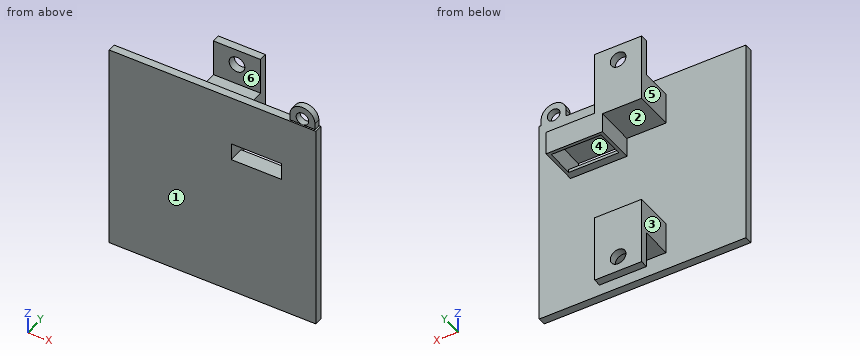
Autodesk Inventor part; units mm, degrees
ref_plane "YZ Plane" through (0, 0, 0) normal (1, 0, 0) x (0, 1, 0)
ref_plane "XZ Plane" through (0, 0, 0) normal (0, 1, 0) x (-1, 0, 0)
ref_plane "XY Plane" through (0, 0, 0) normal (0, 0, 1) x (1, 0, 0)
sketch "Szkic1" plane through (0, 0, 0) normal (0, 1, 0) x (-1, 0, 0)
  line L0 (26.7, -27.1) -> (-26.7, -27.1)
  line L1 (-26.7, -27.1) -> (-26.7, 27.1)
  line L2 (-26.7, 27.1) -> (26.7, 27.1)
  line L3 (26.7, 27.1) -> (26.7, -27.1)
  line L4 (26.7, -27.1) -> (-26.7, 27.1) construction
  line L5 (-26.7, -27.1) -> (26.7, 27.1) construction
  point P0 (0, 0)
  dimension "d0" = 53.4
  dimension "d1" = 54.2
extrude "Wyciągnięcie proste1" add sketch "Szkic1" along normal blind 1.6
sketch "Szkic11" plane through (0, 1.6, 0) normal (0, 1, 0) x (1, 0, 0)
  line L0 (-26.7, -27.1) -> (26.7, -27.1)
  line L1 (26.7, -27.1) -> (25.9, -27.1)
  line L2 (25.9, -27.1) -> (19.5, -27.1)
  line L3 (19.5, -27.1) -> (19.5, -28.7)
  line L4 (19.5, -28.7) -> (25.9, -28.7)
  line L5 (25.9, -28.7) -> (25.9, -27.1)
  arc A0 (19.5, -28.7) -> (25.9, -28.7) centre (22.7, -28.7) ccw
  point P0 (0, 0)
  dimension "d37" = 0.8
  dimension "d38" = 6.4
  dimension "d39" = 1.6
  dimension "d40" = 3.2
extrude "Wyciągnięcie proste10" add sketch "Szkic11" against normal blind 1.6
sketch "Szkic12" plane through (0, 1.6, 0) normal (0, 1, 0) x (1, 0, 0)
  arc A0 (19.5, -28.7) -> (25.9, -28.7) centre (22.7, -28.7) ccw
  circle A1 centre (22.7, -28.7) radius 1.6
  point P0 (0, 0)
  dimension "d43" = 3.2
extrude "Wyciągnięcie proste11" cut sketch "Szkic12" against normal through all
sketch "Szkic24" plane through (0, 1.6, 0) normal (0, 1, 0) x (1, 0, 0)
  line L0 (11.2, -12.1) -> (11.2, -27.1)
  line L1 (-26.7, -27.1) -> (19.5, -27.1)
  line L2 (11.2, -12.1) -> (26.2, -12.1) construction
  line L3 (11.2, -12.1) -> (26.7, -12.1)
  line L4 (26.7, -27.1) -> (26.7, 27.1)
  line L5 (11.2, -12.1) -> (26.7, -12.1) construction
  line L6 (4.8, -9.9) -> (17.6, -9.9)
  line L7 (17.6, -9.9) -> (17.6, -14.3)
  line L8 (17.6, -14.3) -> (4.8, -14.3)
  line L9 (4.8, -14.3) -> (4.8, -9.9)
  line L10 (4.8, -9.9) -> (17.6, -14.3) construction
  line L11 (17.6, -9.9) -> (4.8, -14.3) construction
  point P0 (0, 0)
  dimension "d104" = 15
  dimension "d105" = 90
  dimension "d106" = 15.5
  dimension "d107" = 0
  dimension "d108" = 12.8
  dimension "d109" = 4.4
extrude "Wyciągnięcie proste22" cut sketch "Szkic24" against normal through all
sketch "Szkic33" plane through (0, 1.6, 0) normal (0, 1, 0) x (1, 0, 0)
  line L0 (4.8, -14.3) -> (17.6, -14.3)
  line L1 (4, 4) -> (4, 25.6)
  line L2 (17.6, -14.3) -> (4, -14.3)
  line L3 (4, -14.3) -> (4, -15.1)
  line L4 (4, -15.1) -> (17.6, -15.1)
  line L5 (17.6, -15.1) -> (17.6, -14.3)
  line L6 (4, -15.1) -> (4.8, -15.1)
  line L7 (4.8, -15.1) -> (4.8, -9.1)
  line L8 (4.8, -9.1) -> (4, -9.1)
  line L9 (4, -9.1) -> (4, -15.1)
  line L10 (17.6, -15.1) -> (18.4, -15.1)
  line L11 (18.4, -15.1) -> (18.4, -9.1)
  line L12 (18.4, -9.1) -> (17.6, -9.1)
  line L13 (17.6, -9.1) -> (17.6, -15.1)
  point P0 (0, 0)
  point P1 (4, -21.6)
  point P2 (4, -10)
  point P3 (17.6, -14.3)
  point P4 (4, -10)
  dimension "d139" = 0.8
  dimension "d140" = 6
  dimension "d141" = 0.8
extrude "Wyciągnięcie proste30" add sketch "Szkic33" along normal blind 10
sketch "Szkic34" plane through (0, 1.6, 0) normal (0, 1, 0) x (1, 0, 0)
  line L0 (17.6, -9.9) -> (4.8, -9.9)
  line L1 (4.8, -14.3) -> (4.8, -9.1)
  line L2 (17.6, -9.9) -> (4.8, -9.9)
  line L3 (4.8, -9.9) -> (4.8, -9.1)
  line L4 (4.8, -9.1) -> (17.6, -9.1)
  line L5 (17.6, -9.1) -> (17.6, -9.9)
  point P0 (0, 0)
extrude "Wyciągnięcie proste31" add sketch "Szkic34" along normal blind 2
sketch "Szkic35" plane through (0, 11.6, 0) normal (0, 1, 0) x (1, 0, 0)
  line L0 (4.8, -9.1) -> (4, -9.1)
  line L1 (18.4, -15.1) -> (4, -15.1)
  line L2 (4, -15.1) -> (4, -9.1)
  line L3 (4, -9.1) -> (18.4, -9.1)
  line L4 (18.4, -9.1) -> (18.4, -15.1)
  point P0 (0, 0)
  point P1 (4.8, -9.1)
extrude "Wyciągnięcie proste32" add sketch "Szkic35" against normal blind 0.8
sketch "Szkic49" plane through (26.7, 0, 27.1) normal (1, 0, 0) x (0, 0, -1)
  line L0 (54.2, 0) -> (54.2, 1.6)
  line L1 (0, 0) -> (54.2, 0)
  line L2 (54.2, 0) -> (54.2, 1.6)
  line L3 (54.2, 1.6) -> (0, 1.6)
  line L4 (0, 1.6) -> (0, 0)
  point P0 (27.1, 0)
extrude "Wyciągnięcie proste41" cut sketch "Szkic49" against normal blind 0.3
sketch "Szkic50" plane through (-26.7, 0, -27.1) normal (-1, 0, 0) x (0, 0, 1)
  line L0 (0, 1.6) -> (0, 0)
  line L1 (0, 0) -> (54.2, 0)
  line L2 (0, 1.6) -> (54.2, 1.6)
  line L3 (54.2, 1.6) -> (54.2, 0)
  line L4 (54.2, 0) -> (0, 0)
  line L5 (0, 0) -> (0, 1.6)
  point P0 (27.1, 0)
extrude "Wyciągnięcie proste42" cut sketch "Szkic50" against normal blind 0.3
sketch "Szkic57" plane through (0, 0, 0) normal (0, -1, 0) x (1, 0, 0)
  line L0 (-26.4, -27.1) -> (-26.4, 27.1)
  line L1 (-26.4, 27.1) -> (26.4, 27.1)
  line L2 (26.4, 27.1) -> (26.4, -27.1)
  line L3 (26.4, -27.1) -> (-26.4, -27.1)
  line L4 (-26.4, -27.1) -> (-26.4, 27.1)
  line L5 (4.8, 14.3) -> (17.6, 14.3)
  line L6 (4.8, 9.9) -> (17.6, 9.9)
  line L7 (4.8, 14.3) -> (17.6, 14.3)
  line L8 (17.6, 14.3) -> (17.6, 9.9)
  line L9 (17.6, 9.9) -> (4.8, 9.9)
  line L10 (4.8, 9.9) -> (4.8, 14.3)
  point P0 (0, 0)
  point P1 (17.6, 14.3)
extrude "Wyciągnięcie proste48" add sketch "Szkic57" along normal blind 0.4
sketch "Szkic62" plane through (26.4, 1.6, -27.1) normal (0, 0, -1) x (-1, 0, 0)
  line L0 (52.8, 0) -> (52.8, -2)
  line L1 (52.8, -2) -> (0, -2)
  line L2 (0, -2) -> (0, 0)
  line L3 (0, 0) -> (52.8, 0)
  line L4 (52.8, 0) -> (52.8, -2)
  point P0 (26.4, -1.6)
extrude "Wyciągnięcie proste52" cut sketch "Szkic62" against normal blind 0.4
sketch "Szkic63" plane through (0, 1.6, 0) normal (0, 1, 0) x (1, 0, 0)
  line L0 (0, 0) -> (0, 27.5)
  line L1 (0, 0) -> (27.5, 0) construction
  circle A0 centre (0, 27.5) radius 2
  line L2 (0, 0) -> (0, -27.5)
  line L3 (0, 0) -> (27.5, 0) construction
  circle A1 centre (0, -27.5) radius 2
  dimension "d235" = 27.5
  dimension "d236" = 90
  dimension "d237" = 4
  dimension "d238" = 27.5
  dimension "d239" = 90
  dimension "d240" = 4
sketch "Szkic64" plane through (0, 1.6, 0) normal (0, 1, 0) x (1, 0, 0)
  line L0 (26.4, 26.7) -> (-26.4, 26.7)
  line L1 (0, 26.7) -> (0, 25.1)
  line L2 (0, 25.1) -> (-4, 25.1)
  line L3 (-4, 25.1) -> (-4, 18.7)
  line L4 (-4, 18.7) -> (0, 18.7)
  line L5 (0, 18.7) -> (0, 25.1)
  point P0 (0, 0)
  dimension "d241" = 1.6
  dimension "d242" = 4
  dimension "d243" = 6.4
extrude "Wyciągnięcie proste53" add sketch "Szkic64" along normal blind 8
mirror "Odbij11" about plane through (0, 0, 0) normal (1, 0, 0) of "Wyciągnięcie proste53"
sketch "Szkic65" plane through (0, 9.6, 0) normal (0, 1, 0) x (1, 0, 0)
  line L0 (-4, 25.1) -> (4, 25.1)
  line L1 (-4, 25.1) -> (4, 25.1)
  line L2 (4, 25.1) -> (4, 31.5)
  line L3 (4, 31.5) -> (-4, 31.5)
  line L4 (-4, 31.5) -> (-4, 25.1)
  point P0 (0, 0)
  dimension "d246" = 6.4
extrude "Wyciągnięcie proste54" add sketch "Szkic65" along normal blind 2
mirror "Odbij12" about plane through (0, 0, 0) normal (0, 0, 1) of "Wyciągnięcie proste53", "Odbij11", "Wyciągnięcie proste54"
extrude "Wyciągnięcie proste55" cut sketch "Szkic63" along normal through all
sketch "Szkic66" plane through (0, 9.6, 0) normal (0, 1, 0) x (1, 0, 0)
  line L0 (-4, 18.7) -> (-4, 25.1)
  line L1 (-4, 25.1) -> (4, 25.1)
  line L2 (-4, 18.7) -> (4, 18.7)
  line L3 (4, 18.7) -> (4, 25.1)
  line L4 (4, 25.1) -> (-4, 25.1)
  line L5 (-4, 25.1) -> (-4, 18.7)
  line L6 (-4, -25.1) -> (-4, -18.7)
  line L7 (-4, -25.1) -> (4, -25.1)
  line L8 (-4, -18.7) -> (4, -18.7)
  line L9 (4, -18.7) -> (4, -25.1)
  line L10 (4, -25.1) -> (-4, -25.1)
  line L11 (-4, -25.1) -> (-4, -18.7)
  point P0 (0, 0)
extrude "Wyciągnięcie proste56" add sketch "Szkic66" along normal blind 2
sketch "Szkic67" plane through (4, 1.6, -25.1) normal (0, 0, -1) x (-1, 0, 0)
  line L0 (0, 8) -> (8, 8)
  line L1 (8, 0) -> (0, 0)
  line L2 (8, 8) -> (0, 8)
  line L3 (0, 8) -> (0, 0)
  line L4 (0, 0) -> (8, 0)
  line L5 (8, 0) -> (8, 8)
  point P0 (4, -1.6)
extrude "Wyciągnięcie proste57" cut sketch "Szkic67" against normal blind 3
sketch "Szkic68" plane through (-4, 1.6, -18.7) normal (0, 0, 1) x (1, 0, 0)
  line L0 (8, 0) -> (8, 10)
  line L1 (8, 0) -> (0, 0)
  line L2 (8, 10) -> (0, 10)
  line L3 (0, 10) -> (0, 0)
  line L4 (0, 0) -> (8, 0)
  line L5 (8, 0) -> (8, 10)
  point P0 (4, -1.6)
extrude "Wyciągnięcie proste58" add sketch "Szkic68" along normal blind 4.6
sketch "Szkic69" plane through (-4, 9.6, -31.5) normal (-1, 0, 0) x (0, 0, 1)
  line L0 (17.4, 2) -> (17.4, -8)
  line L1 (17.4, 2) -> (17.4, -8)
  line L2 (9.4, -8) -> (17.4, -8)
  line L3 (17.4, -8) -> (9.4, -8)
  line L4 (9.4, -8) -> (9.4, 0)
  line L5 (9.4, -8) -> (9.4, 0)
  line L6 (0, 0) -> (0, 2)
  line L7 (9.4, 0) -> (0, 0)
  line L8 (0, 0) -> (0, 2)
  line L9 (0, 2) -> (17.4, 2)
  line L10 (0, 2) -> (17.4, 2)
  point P0 (31.5, -9.6)
extrude "Wyciągnięcie proste59" add sketch "Szkic69" along normal blind 2
mirror "Odbij13" about plane through (0, 0, 0) normal (1, 0, 0) of "Wyciągnięcie proste59"
mirror "Odbij14" about plane through (0, 0, 0) normal (0, 0, 1) of "Wyciągnięcie proste56", "Wyciągnięcie proste57", "Wyciągnięcie proste58", "Wyciągnięcie proste59", "Odbij13"
sketch "Szkic70" plane through (4.8, 1.6, 14.3) normal (0, -1, 0) x (1, 0, 0)
  line L0 (0, -0.2) -> (1.2, -0.2)
  line L1 (1.2, -0.2) -> (0, -0.2)
  line L2 (0, -0.2) -> (0, 0)
  line L3 (0, 0) -> (1.2, 0)
  line L4 (1.2, 0) -> (1.2, -0.2)
  point P0 (-4.8, -14.3)
extrude "Wyciągnięcie proste60" cut sketch "Szkic70" against normal up to surface (9.2 mm away)
properties part number "uchwyt2"
Can you work these out from the model? Positions are in its coordinate system, mm. Face numbers are marked on the shaded views. A direction names the side the tool comes from. Coordinates: 2 decimals unless noted, no trailing zeros. Loops run counter-clockwise (first coordinate to the right, second up) from the corner with the lowest first, then second, coordinate; pieces in that order, holes last. Notation, with made-up numbers: (61.25, 61) - (107.25, 61) arc R19 cw to (107.25, 83) - close; hole circle Ø2 at (38, 44). An arc over 180 degrees is marked (long way). Use a Markdown table: item, result.
Item 1: I want a section at A-A on y = 2.75. Please give me the cut outline in (x, z), and give its area (3 significant figures).
Numbers:
| item | result |
|---|---|
| outline | (-6, -22.1) - (6, -22.1) - (6, -14.1) - (-6, -14.1) - close; (-6, 14.1) - (4, 14.1) - (4, 9.1) - (18.4, 9.1) - (18.4, 15.1) - (6, 15.1) - (6, 22.1) - (-6, 22.1) - close; hole (4.8, 9.9) - (17.6, 9.9) - (17.6, 14.3) - (4.8, 14.3) - close |
| area | 220 mm2 |
Item 2: For the marked faces 1, 2 and 3, which set-ups out of +Z, -Z, +X, -X, +Y, -Y let a thin tool reach every point of the face, with its end or its side?
Numbers:
| item | result |
|---|---|
| face 1 | +Z, -Z, +X, -X, -Y |
| face 2 | -X, +Y |
| face 3 | +Z, -Z, -X, +Y |
Item 3: Will these pins go through, and if not, where does the flat tip stop? pin 1 (2.5 mm diameter, centred on y = 8, z = 11, fed in from -X); pin 2 (2 mm diameter, centred on x = -15.5, y = 1.5, fed in from +Z); pin 3 (1.6 mm diameter, centred on x = -13, y = 0.5, fed in from -Z).
Numbers:
| item | result |
|---|---|
| pin 1 | stops at x = 4 |
| pin 2 | stops at z = 27.1 |
| pin 3 | stops at z = -26.7 |
Item 4: I want a section at C-C on x = 0. Please give me the cut outline in (y, z), and give its area (3 significant figures).
Numbers:
| item | result |
|---|---|
| outline | (-0.4, -26.7) - (1.6, -26.7) - (1.6, -22.1) - (9.6, -22.1) - (9.6, -25.5) - (11.6, -25.5) - (11.6, -14.1) - (1.6, -14.1) - (1.6, 14.1) - (11.6, 14.1) - (11.6, 25.5) - (9.6, 25.5) - (9.6, 22.1) - (1.6, 22.1) - (1.6, 27.1) - (-0.4, 27.1) - close; (9.6, -31.5) - (11.6, -31.5) - (11.6, -29.5) - (9.6, -29.5) - close; (9.6, 29.5) - (11.6, 29.5) - (11.6, 31.5) - (9.6, 31.5) - close |
| area | 289 mm2 |
Item 5: I want a section at D-D on x = 16. Please give me the cut outline in (y, z), and give its area (3 significant figures).
Numbers:
| item | result |
|---|---|
| outline | (-0.4, -26.7) - (1.6, -26.7) - (1.6, 9.1) - (3.6, 9.1) - (3.6, 9.9) - (-0.4, 9.9) - close; (-0.4, 14.3) - (10.8, 14.3) - (10.8, 9.1) - (11.6, 9.1) - (11.6, 15.1) - (1.6, 15.1) - (1.6, 27.1) - (-0.4, 27.1) - close |
| area | 113 mm2 |
Item 6: If I drill on probe 1 along Z at (x, y) = (0, 10.6); probe 2 along X at (y, z) = (0.4, 28.7); probe 3 along Z at (x, y) = (0, 6), over which ranges is the centre line in solid material (lowest first)? Write a range as from..to.
Numbers:
| item | result |
|---|---|
| probe 1 | z = -31.5..-29.5, -25.5..-14.1, 14.1..25.5, 29.5..31.5 |
| probe 2 | x = 19.5..21.1, 24.3..25.9 |
| probe 3 | z = -22.1..-14.1, 14.1..22.1 |
Item 7: We'd pull the mould along X, two halves only. Please class the marked faces 4, 5 and 6: released by +X, released by -X, zero draft, split by the parting line, or undercut.
Numbers:
| item | result |
|---|---|
| face 4 | undercut |
| face 5 | released by -X |
| face 6 | zero draft |
Item 8: I want a section at B-B on z = -27.5. Please give me the cut outline in (x, y), and give its area (3 significant figures).
Numbers:
| item | result |
|---|---|
| outline | (-6, 9.6) - (-2, 9.6) - (-2, 11.6) - (-6, 11.6) - close; (2, 9.6) - (6, 9.6) - (6, 11.6) - (2, 11.6) - close |
| area | 16.0 mm2 |
